```python
from build123d import *

# Parameters (mm, degrees)
F1_DEPTH      = 15.1
F1_DEPTH_BACK = 15.1
F2_DEPTH      = 2.5
F2_DEPTH_BACK = 2.5
F3_W          = 14
F3_H          = 1
F4_DEPTH      = 2
F4_DEPTH_BACK = 4
F6_DEPTH      = 1.5
F7_W          = 5.0940940584
F7_H          = 2
F7_W_2        = 5.0823323011
F7_W_3        = 5.0705705438
F7_W_4        = 5.0588087865
F7_W_5        = 5.0470470292
F7_W_6        = 5.0352852719
F7_W_7        = 5.0235235146
F7_W_8        = 5.0117617573
F7_W_9        = 5
F8_DEPTH      = 6.501
F10_DEPTH     = 15
F11_R         = 12


with BuildPart() as f1:
    # F0 (on Front) → F1 (new body, two sides)
    with BuildSketch(Plane.XZ) as f1_sk:
        with BuildLine():
            Line((-71.4607020907, 40.6989861274), (-71.4607020907, 38.1989861274))
            Line((-71.4607020907, 38.1989861274), (-31.4607020907, 38.1989861274))
            Line((-31.4607020907, 38.1989861274), (-25.4607020907, 35.1989861274))
            ThreePointArc((-25.4607020907, 35.1989861274), (-28.2968833209, 38.1276975126), (-31.4607020907, 40.6989861274))
            Line((-31.4607020907, 40.6989861274), (-71.4607020907, 40.6989861274))
        make_face()
    extrude(amount=F1_DEPTH)
    extrude(f1_sk.sketch, amount=-F1_DEPTH_BACK)

    # F0 (on Front) → F2 (join, two sides)
    with BuildSketch(Plane.XZ) as f2_sk:
        with BuildLine():
            Line((-71.4607020907, 36.4489861274), (-71.4607020907, 38.1989861274))
            Line((-71.4607020907, 38.1989861274), (-71.4607020907, 40.6989861274))
            Line((-71.4607020907, 40.6989861274), (-72.2107020907, 40.6989861274))
            ThreePointArc((-72.2107020907, 40.6989861274), (-72.387478786, 40.6257628227), (-72.4607020907, 40.4489861274))
            Line((-72.4607020907, 40.4489861274), (-72.4607020907, 35.9489861274))
            ThreePointArc((-72.4607020907, 35.9489861274), (-72.387478786, 35.7722094321), (-72.2107020907, 35.6989861274))
            Line((-72.2107020907, 35.6989861274), (-71.2107020907, 35.6989861274))
            ThreePointArc((-71.2107020907, 35.6989861274), (-71.0339253954, 35.7722094321), (-70.9607020907, 35.9489861274))
            Line((-70.9607020907, 35.9489861274), (-70.9607020907, 36.1989861274))
            Line((-70.9607020907, 36.1989861274), (-71.2107020907, 36.1989861274))
            ThreePointArc((-71.2107020907, 36.1989861274), (-71.387478786, 36.2722094321), (-71.4607020907, 36.4489861274))
        make_face()
    extrude(amount=F2_DEPTH)
    extrude(f2_sk.sketch, amount=-F2_DEPTH_BACK)

    # F7 (on face) → F8 (cut, through all)
    with BuildSketch(Plane.XY.offset(40.6989861274)):
        Polygon((-31.4607020907, -10.9998155474), (-31.4607020907, -12.9998155474), (-23.5907521141, -12.9998155474), (-23.6532528544, -10.9998155474), align=None)
        Polygon((-31.4607020907, -7.999838604), (-31.4607020907, -9.999838604), (-23.6025138714, -9.999838604), (-23.6650146117, -7.999838604), align=None)
        Polygon((-23.676776369, -4.9998616605), (-31.4607020907, -4.9998616605), (-31.4607020907, -6.9998616605), (-23.6142756287, -6.9998616605), align=None)
        Polygon((-23.6885381263, -1.9998847171), (-31.4607020907, -1.9998847171), (-31.4607020907, -3.9998847171), (-23.626037386, -3.9998847171), align=None)
        Polygon((-23.7002998836, 1.0000922263), (-31.4607020907, 1.0000922263), (-31.4607020907, -0.9999077737), (-23.6377991433, -0.9999077737), align=None)
        Polygon((-23.7120616409, 4.0000691697), (-31.4607020907, 4.0000691697), (-31.4607020907, 2.0000691697), (-23.6495609006, 2.0000691697), align=None)
        Polygon((-23.7238233982, 7.0000461132), (-31.4607020907, 7.0000461132), (-31.4607020907, 5.0000461132), (-23.6613226579, 5.0000461132), align=None)
        Polygon((-23.7355851555, 10.0000230566), (-31.4607020907, 10.0000230566), (-31.4607020907, 8.0000230566), (-23.6730844152, 8.0000230566), align=None)
        Polygon((-23.6848461725, 11), (-23.7473469128, 13), (-31.4607020907, 13), (-31.4607020907, 11), align=None)
        with Locations((-34.0077491199, 12)):
            Rectangle(F7_W, F7_H)
        with Locations((-34.0018682413, 9.0000230566)):
            Rectangle(F7_W_2, F7_H)
        with Locations((-33.9959873626, 6.0000461132)):
            Rectangle(F7_W_3, F7_H)
        with Locations((-33.990106484, 3.0000691697)):
            Rectangle(F7_W_4, F7_H)
        with Locations((-33.9842256053, 9.22263e-05)):
            Rectangle(F7_W_5, F7_H)
        with Locations((-33.9783447267, -2.9998847171)):
            Rectangle(F7_W_6, F7_H)
        with Locations((-33.972463848, -5.9998616605)):
            Rectangle(F7_W_7, F7_H)
        with Locations((-33.9665829694, -8.999838604)):
            Rectangle(F7_W_8, F7_H)
        with Locations((-33.9607020907, -11.9998155474)):
            Rectangle(F7_W_9, F7_H)
    extrude(amount=-F8_DEPTH, mode=Mode.SUBTRACT)

    # F11
    f11_edges = [f1.edges().sort_by_distance(p)[0] for p in [
        (-71.460702, -15.1, 39.448986),
        (-71.460702, 15.1, 39.448986),
    ]]
    fillet(f11_edges, radius=F11_R)



with BuildPart() as f4:
    # F3 (on face) → F4 (new body, two sides)
    with BuildSketch(Plane(origin=(0, 0, 38.1989861274), x_dir=(1, 0, 0), z_dir=(0, 0, -1))) as f4_sk:
        with Locations((-43.4607020907, -15.6)):
            Rectangle(F3_W, F3_H)
    extrude(amount=-F4_DEPTH)
    extrude(f4_sk.sketch, amount=F4_DEPTH_BACK)

    # F5 (on face) → F6 (join)
    with BuildSketch(Plane.XZ.offset(-15.1)):
        Polygon((-36.4607020907, 34.1989861274), (-36.4607020907, 35.9489861274), (-43.4607020907, 35.9489861274), (-44.4607020907, 34.1989861274), align=None)
        Polygon((-44.4607020907, 34.1989861274), (-43.4607020907, 35.9489861274), (-50.4607020907, 35.9489861274), (-50.4607020907, 34.1989861274), align=None)
    extrude(amount=F6_DEPTH)

    # F9 (on face) → F10 (cut)
    with BuildSketch(Plane(origin=(-50.4607020907, 0, 0), x_dir=(0, -1, 0), z_dir=(-1, 0, 0))):
        Polygon((-15.1, 35.9489861274), (-13.6, 35.8239861274), (-13.6, 35.9489861274), align=None)
        Polygon((-13.6, 35.0739861274), (-15.1, 34.9489861274), (-13.6, 34.9489861274), align=None)
        Polygon((-15.1, 34.9489861274), (-16.1, 34.9489861274), (-16.1, 34.1989861274), (-13.6, 34.1989861274), (-13.6, 34.9489861274), align=None)
    extrude(amount=-F10_DEPTH, mode=Mode.SUBTRACT)


with BuildPart() as f1_1:
    add(f1.part)

    add(f4.part)  # F12 merges F4
    # F12: F4 across plane
    add(f4.part.mirror(Plane.XZ))


solid = f1_1.part
```
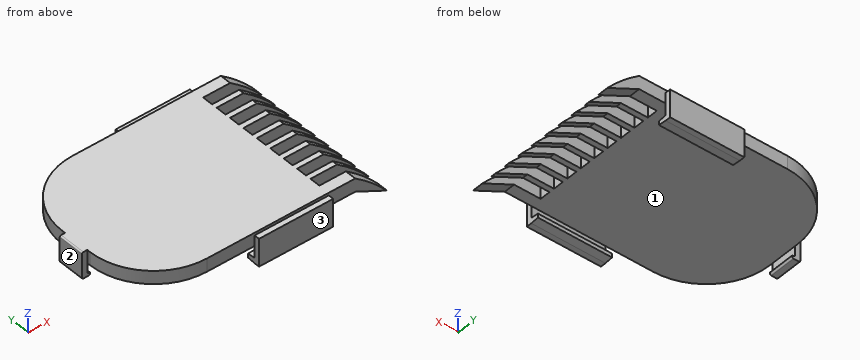
CAD build for the part. Positions are in the model's coordinates, mm. Face numbers are marked on the shaded views. Round coordinates to 2 decimals unless told otherwise and drop trailing zeros. Order: outer loops, then holes, each group sorted by start corner. A loop starts at its lowest first (then second) coordinate and runs counter-clockwise, first axis right, second up. Notation, with made-up numbers: (31.5, 39.25) - (69.5, 39.25) arc R27 cw to (69.5, 77.25) - close; hole circle Ø4 at (89, 9). An arc over 180 degrees is marked (long way). Answer in a Markdown table with one row per item. Add a question column.
(1) Mould opens along Y. For the marked faces 1, 2 and 3 say: +Y half, -Y half, draft (parallel to the pull), parting line (faces both ways), or undercut.
(2) Drop flat-ended pins along their axis: pin 1 Ø5 at (x, y) = (-56, 3) entering from -Z; pin 2 Ø3 at (x, z) = (-28.5, 39) entering from +Y; pin 3 Ø1.6 at (x, z) = (-31.5, 36.5) entering from -Y; pin 4 Ø3 at (x, z) = (-29, 37.5) entering from -Y. Give the stop position or say it passes through.
(3) Probe L1, parallel to Y at x = -38, z = 37.7; L2, parallel to Y at x = -40, z = 35.6; L3, parallel to Z at x = -68.5, y = -4.5. List the from-to ranges inside material, lowest first. Write a range as [from, to].
(4) Band-saw the part on A-A on x = -33. Count the separate pieces of the cut face and the enclosed holes in it, and give its area (3 significant figures).
(5) Band-saw the part on D-D on x = -56. List the corners of the cut face in (y, z).
(6) Band-saw the part on C-C on y = -10.5. List the corners of the cut face in (x, z).
Data:
| question | item | result |
|---|---|---|
| 1 | face 1 | undercut |
| 1 | face 2 | draft |
| 1 | face 3 | -Y half |
| 2 | pin 1 | stops at z = 38.2 |
| 2 | pin 2 | stops at y = 15.1 |
| 2 | pin 3 | passes through |
| 2 | pin 4 | stops at y = -15.1 |
| 3 | L1 | y = [-16.1, -15.1], [15.1, 16.1] |
| 3 | L2 | y = [-16.1, -13.6], [13.6, 16.1] |
| 3 | L3 | z = [38.2, 40.7] |
| 4 | separate pieces | 10 |
| 4 | enclosed holes | 0 |
| 4 | area | 30.5 mm^2 |
| 5 | outline | (-15.1, 38.2) - (15.1, 38.2) - (15.1, 40.7) - (-15.1, 40.7) - close |
| 6 | outline | (-68.91, 38.2) - (-31.46, 38.2) - (-25.46, 35.2) arc R34.28 ccw to (-31.46, 40.7) - (-68.91, 40.7) - close |
